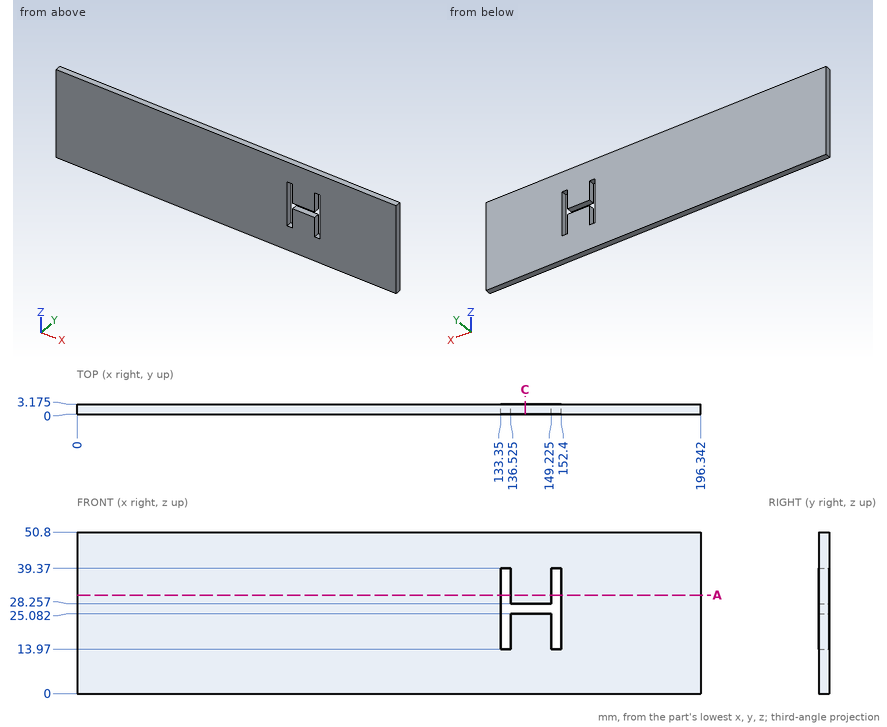
Source: three-view drawing plus pictorial views. Frame: mm from the lowest corner of the part. Give positions to 0.01 mm unless a question says otherwise; leave off trailing zeros. Loops run counter-clockwise (first coordinate to the right, second up) from the corner with the lowest first, then second, coordinate; pieces in that order, holes last. Notation, with made-up numbers: (88.25, 57) -> (130.25, 57) arc R19 cw to (130.25, 74) -> close; hole circle Ø4 at (44.25, 43.25). An arc over 180 degrees is marked (long way). Put each result on its own line as item: value. Start each with the question number.
1) Material intervals for probe 1 along X at (y, z) = (1.3, 27); probe 2 along Z at (x, y) = (140, 1.1); probe 3 along Z at (x, y) = (133.5, 2.1), sorted ascending.
2) Cut plane C-C (x = 141). Return loops of the section in (y, z) (1 decimal).
3) Cut plane A-A (z = 31). State how many separate pieces and enclosed holes the cut face has.
Results are:
1. probe 1: x = 0 to 133.35, 152.4 to 196.34
1. probe 2: z = 0 to 25.08, 28.26 to 50.8
1. probe 3: z = 0 to 13.97, 39.37 to 50.8
2. outline: (0, 0) -> (3.2, 0) -> (3.2, 25.1) -> (0, 25.1) -> close; (0, 28.3) -> (3.2, 28.3) -> (3.2, 50.8) -> (0, 50.8) -> close
3. separate pieces: 3
3. enclosed holes: 0
